Build history of the part. All positions in model axes, mm. Face numbers are marked on the shaded views. Give positions to 0.01 mm unless a question says otherwise; leave off trailing zeros. Loops run counter-clockwise (first coordinate to the right, second up) from the corner with the lowest first, then second, coordinate; pieces in that order, holes last. Notation, with made-up numbers: (-9.75, -11.75) -> (-4.75, -11.75) arc R19 ccw to (-4.75, 2.25) -> close; hole circle Ø7 at (57, 11.25). An arc over 180 degrees is marked (long way). Answer as a JSON object with one key per item and string values. Group by question number.
Q1. Two-plate mould, pull along Z, no slides. Class the marked faces 1 and 2: pulls with the +Z half, pulls with the -Z half, needs draft (parallel to the pull), parting line crosses it, or undercut.
Q2. Wall check: probe 1 along X at (y, z) = (2, 0); probe 2 along X at (y, z) = (1.25, -0.9). Give the ranges that are in metal, low to high. Write a range as from..to.
Q3. Band-saw the part on C-C, the plane y = 5.75. Write the cut outline in (x, z).
from build123d import *

# Parameters (mm, degrees)
SKETCH1_R           = 1.25
SKETCH1_R_2         = 1
BOSS_EXTRUDE1_DEPTH = 10
FILLET1_R           = 0.01


with BuildPart() as part:
    # Sketch1 → Boss-Extrude1 (new body)
    with BuildSketch(Plane(origin=(0, 0, 0), x_dir=(1, 0, 0), z_dir=(0, 1, 0))):
        Circle(SKETCH1_R)
        Circle(SKETCH1_R_2, mode=Mode.SUBTRACT)
    extrude(amount=BOSS_EXTRUDE1_DEPTH)

    # Fillet1
    fillet1_edges = [part.edges().sort_by_distance(p)[0] for p in [
        (-1.25, 10, 0),
        (-1, 0, 0),
        (-1, 10, 0),
    ]]
    fillet(fillet1_edges, radius=FILLET1_R)


solid = part.part
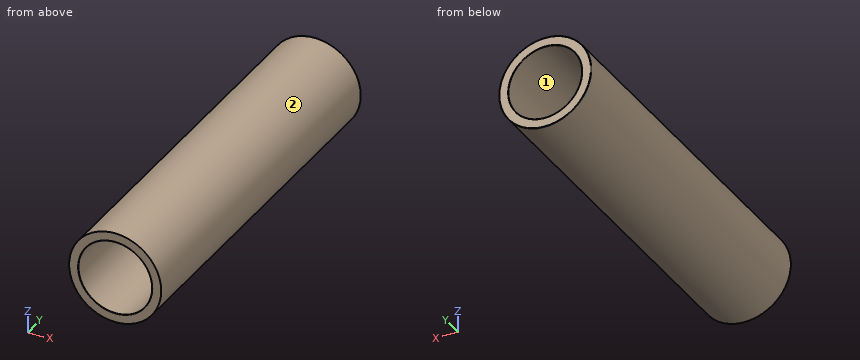
Worked answers:
{
 "1": {"face 1": "undercut", "face 2": "parting line crosses it"},
 "2": {"probe 1": "-1.25..-1, 1..1.25", "probe 2": "-0.87..-0.44, 0.44..0.87"},
 "3": {"outline": "circle Ø2.5 at (0, 0); hole circle Ø2 at (0, 0)"}
}
